```python
from build123d import *

# Parameters (mm, degrees)
EXTRUDE_562_REACH = 36.438
SKETCH_2_R        = 5.773502692
FILLET_616_R      = 1
CHAMFER_1_SIZE    = 1.0735375
FILLET_2_R        = 0.1


with BuildPart() as part:
    # 草圖1 → Revolve 435 (revolve)
    with BuildSketch(Plane.XY, mode=Mode.PRIVATE) as revolve_435_sk:
        Polygon((-2.066666667, 0), (20, 0), (20, 6), (4.3, 6), (3.2263625, 6), (0, 6), (0, 9), (-12, 9), (-12, 5.773502692), (-5.4, 5.773502692), align=None)
    revolve(revolve_435_sk.sketch.rotate(Axis((-2.066666667, 0, 0), (1, 0, 0)), 180), axis=Axis((-2.066666667, 0, 0), (1, 0, 0)))

    # 草圖2 → Extrude 562 (add, up to next)
    with BuildSketch(Plane.ZY.offset(12), mode=Mode.PRIVATE) as extrude_562_sk1:
        Circle(SKETCH_2_R)
    extrude_562_tool1 = extrude(extrude_562_sk1.sketch, amount=-EXTRUDE_562_REACH, mode=Mode.PRIVATE) - part.part
    # 草圖2 → Extrude 562 (add, up to next)
    with BuildSketch(Plane.ZY.offset(12), mode=Mode.PRIVATE) as extrude_562_sk2:
        Polygon((5.773502692, 0), (2.886751346, -5), (-2.886751346, -5), (-5.773502692, 0), (-2.886751346, 5), (2.886751346, 5), align=None)
    extrude_562_tool2 = extrude(extrude_562_sk2.sketch, amount=-EXTRUDE_562_REACH, mode=Mode.PRIVATE) - part.part
    add(extrude_562_tool1.solids().sort_by_distance((-12, 0, 0))[0])
    add(extrude_562_tool2.solids().sort_by_distance((-12, 0, 0))[0])

    # Fillet 616
    fillet_616_edges = [part.edges().sort_by_distance(p)[0] for p in [
        (-12, 9, 0),
    ]]
    fillet(fillet_616_edges, radius=FILLET_616_R)

    # 倒角1
    chamfer_1_edges = [part.edges().sort_by_distance(p)[0] for p in [
        (20, 6, 0),
    ]]
    chamfer(chamfer_1_edges, length=CHAMFER_1_SIZE)

    # 圓角2
    fillet_2_edges = [part.edges().sort_by_distance(p)[0] for p in [
        (0, 6, 0),
    ]]
    fillet(fillet_2_edges, radius=FILLET_2_R)


solid = part.part
```
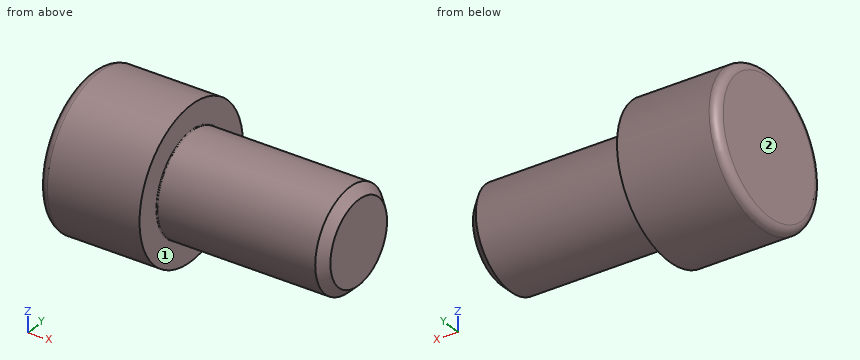
CAD build for the part. Positions are in the model's coordinates, mm. Face numbers are marked on the shaded views. A direction names the side the tool comes from. Coordinates: 2 decimals unless noted, no trailing zeros. Order: outer loops, then holes, each group sorted by start corner. A loop starts at its lowest first (then second) coordinate and runs counter-clockwise, first axis right, second up. Notation, with made-up numbers: (45.5, 69.25) - (58.5, 69.25) arc R18 ccw to (58.5, 83.25) - close; hole circle Ø3 at (43.5, 39.25). An arc over 180 degrees is marked (long way). Answer in a Markdown table with one row per item.
1. Slice it at A-A, the plane y = 0. List the corners of the cut face in (x, z).
Answer:
| item | result |
|---|---|
| outline | (-12, -8) arc R1 ccw to (-11, -9) - (0, -9) - (0, -6.1) arc R0.1 cw to (0.1, -6) - (18.93, -6) - (20, -4.93) - (20, 4.93) - (18.93, 6) - (0.1, 6) arc R0.1 cw to (0, 6.1) - (0, 9) - (-11, 9) arc R1 ccw to (-12, 8) - close |
2. Drill centre lines: L1, parallel to Z at x = 11, y = -0.25; L2, parallel to X at y = -6.5, z = 1.5; L3, parallel to Y at x = -5, z = 3. Where is each one in solid material? Low to high. Write a range as from..to.
Answer:
| item | result |
|---|---|
| L1 | -5.99..5.99 |
| L2 | -12..0 |
| L3 | -8.49..8.49 |
3. Slice it at D-D, the plane x = 14. List the corners of the cut face in (y, z).
Answer:
| item | result |
|---|---|
| outline | circle Ø12 at (0, 0) |
4. Flat gauge pins, fed straight in: P1, Ø8, axis at x = 7, z = 6, coming from the +Y side; P2, Ø1.5, axis at x = 14.5, y = 0.5, coming from the -Z side; P3, Ø2, axis at x = -4.5, y = -6.5, coming from the +Z side. Where does each tip first touch, or does it go through?
Answer:
| item | result |
|---|---|
| P1 | y = 5.66 |
| P2 | z = -6 |
| P3 | z = 7.12 |
5. Slice it at C-C, the plane x = -2. List the corners of the cut face in (y, z), then the cut area to 3 significant figures.
Answer:
| item | result |
|---|---|
| outline | circle Ø18 at (0, 0) |
| area | 254 mm² |
6. 3-axis set-ups, long thin cutter, end or side, ignore diameter. For the marked faces 1 and 2: which of +Z, -Z, +X, -X, +Y, -Y reach the whole face in a straight line?
Answer:
| item | result |
|---|---|
| face 1 | +X |
| face 2 | +Z, -Z, -X, +Y, -Y |
